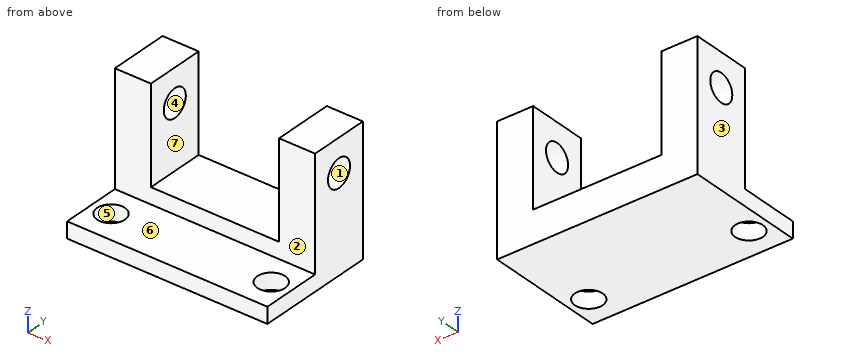
```python
from build123d import *

# Parameters (mm, degrees)
F0_W     = 31.75
F0_H     = 19.05
F1_DEPTH = 20.32
F2_W     = 31.75
F2_H     = 9.525
F3_DEPTH = 17.78
F4_W     = 20.32
F4_H     = 9.525
F5_DEPTH = 15.24
F7_D     = 4.4
F9_D     = 4.4


with BuildPart() as f1:
    # F0 (on Top) → F1 (new body)
    with BuildSketch(Plane.XY):
        with Locations((15.875, 9.525)):
            Rectangle(F0_W, F0_H)
    extrude(amount=F1_DEPTH)

    # F2 (on face) → F3 (cut)
    with BuildSketch(Plane.XY.offset(20.32)):
        with Locations((15.875, 4.7625)):
            Rectangle(F2_W, F2_H)
    extrude(amount=-F3_DEPTH, mode=Mode.SUBTRACT)

    # F4 (on face) → F5 (cut)
    with BuildSketch(Plane.XY.offset(20.32)):
        with Locations((15.875, 14.2875)):
            Rectangle(F4_W, F4_H)
    extrude(amount=-F5_DEPTH, mode=Mode.SUBTRACT)

    # F7 (through all)
    with Locations(Plane.XY.offset(2.54)):
        with Locations((3.175, 4.7625), (28.575, 4.7625)):
            Hole(F7_D / 2)

    # F9 (through all)
    with Locations(Plane.YZ.offset(31.75)):
        with Locations((14.2875, 15.08)):
            Hole(F9_D / 2)


solid = f1.part
```
Input: part model. Units: mm. Frame: model coordinates. Face numbers are marked on the shaded views. A direction names the side the tool comes from. Round coordinates to 2 decimals unless told otherwise and drop trailing zeros. Loops run counter-clockwise (first coordinate to the right, second up) from the corner with the lowest first, then second, coordinate; pieces in that order, holes last. Notation, with made-up numbers: M 50.25,-17 L 95.25,-17 A17 ccw 95.25,-1 Z; hole C 4,5.25 d7. An arc over 180 degrees is marked long. Answer in a Markdown table with one row per item. Add a question column.
1. Section A-A (x = 29.5). Give the number of separate pieces and of enclosed holes in the cut face, and give its area (3 significant figures).
2. Contact query for flat-ended pins moving along their axis: pin 1 (5 mm diameter, centred on x = 18.5, y = 4, fed in from +Z); pin 2 (5 mm diameter, centred on y = 7.5, z = 4, fed in from +X); pin 3 (2.5 mm diameter, centred on y = 14.29, z = 15.08, fed in from +X); pin 4 (7.5 mm diameter, centred on x = 14.5, y = 16, fed in from +Z). Output: stop coordinate, or through.
3. Mould query, pull axis Y, two halves, no side actions, for the marked faces 1, 2, 3 and 4. Classes: released by +Y, released by -Y, zero draft, split by the parting line, or undercut.
4. Set-up query: the marked faces 5, 6 and 7. Return all of +Z, -Z, +X, -X, +Y, -Y with unobstructed straight access to the full face (end or side cutting, diameter ignored); none if empty.
5. Ray query, probe 1 along X at (y, z) = (6.5, 2); probe 2 along X at (y, z) = (17.75, 13.5) (3 decimals); probe 3 along Z at (x, y) = (22, 14.5). Return the intervals inside material, ascending.
6. Section C-C (y = 14.25). Output: boundary loops of the cut face in (x, z) (3 decimals).
Values follow:
| question | item | result |
|---|---|---|
| 1 | separate pieces | 2 |
| 1 | enclosed holes | 1 |
| 1 | area | 192 mm^2 |
| 2 | pin 1 | z = 2.54 |
| 2 | pin 2 | x = 31.75 |
| 2 | pin 3 | through |
| 2 | pin 4 | z = 5.08 |
| 3 | face 1 | undercut |
| 3 | face 2 | released by -Y |
| 3 | face 3 | zero draft |
| 3 | face 4 | undercut |
| 4 | face 5 | +Z, -Z |
| 4 | face 6 | +Z, +X, -X, -Y |
| 4 | face 7 | +Z, +Y, -Y |
| 5 | probe 1 | 0 to 1.83, 4.52 to 27.23, 29.92 to 31.75 |
| 5 | probe 2 | 0 to 5.715, 26.035 to 31.75 |
| 5 | probe 3 | 0 to 5.08 |
| 6 | outline | M 0,0 L 31.75,0 L 31.75,12.88 L 26.035,12.88 L 26.035,5.08 L 5.715,5.08 L 5.715,12.88 L 0,12.88 Z; M 0,17.28 L 5.715,17.28 L 5.715,20.32 L 0,20.32 Z; M 26.035,17.28 L 31.75,17.28 L 31.75,20.32 L 26.035,20.32 Z |
